Read the model definition and answer for the solid it produces. Units are mm, in the model's axes. A direction names the side the tool comes from. Coordinates: 2 decimals unless noted, no trailing zeros. Loops run counter-clockwise (first coordinate to the right, second up) from the corner with the lowest first, then second, coordinate; pieces in that order, holes last. Notation, with made-up numbers: (19.25, 14.25) -> (42.25, 14.25) arc R13 cw to (42.25, 20.25) -> close; hole circle Ø2 at (30.5, 49). An arc over 180 degrees is marked (long way). Answer as a JSON object with one key per item and string values. Group by question number.
Q1. Determine the mould class of faces 5 (the flat face through (25.441, 0, -11)), 6 (the cylindrical face through (-16.31, -20.796, 15.284)), 7 (the flat face through (137, -11.112, 9)) for opening direction X: released by +X, released by -X, zero draft, split by the parting line, or undercut.
Q2. Straight lines are drawn through the part: line 1 along Z through (x, y) = (0, 22); line 2 along X through (y, z) = (-24, -9); line 3 along X through (y, z) = (-17, 0.5). For each, find the intervals that lie inside material, in ascending order. Write a range as [from, to].
Q3. The part is cut by section B-B on z = -4. Write down the section's boundary in (x, y), and give its area (3 significant figures).
Q4. The part is cut by section D-D on z = -20. Write down the section's boundary in (x, y), and give its area (3 significant figures).
Q5. The part is cut by section C-C on y = 21.5. Write down the section's boundary in (x, z), and give its area (3 significant figures).
Q6. Each of these flat-tipped pins is pushed along its axis until it touches: P1, Ø10, axis at y = -17.5, z = -6, coming from the -X side; P2, Ø24.5, axis at y = -1.5, z = -16.5, coming from the -X side; P3, Ø3, axis at y = -16.5, z = 17.5, coming from the -X side; P4, Ø15, axis at x = 0, z = 0, coming from the +Y side. Where does it stop, or does it pass through?
Q7. The part is cut by section A-A on y = -13.5. Write down the section's boundary in (x, z).
Q8. For faces 1 (the flat face through (12, -11.163, -5)), 2 (the flat face through (107, 6, 0)), 3 (the flat face through (112.166, -21, -11)), 4 (the flat face through (150.089, -21, 11)), determine the directions among +Z, -Z, +X, -X, +Y, -Y from which every point of the face is accessible in a straight line to the end or side of a thin tool.
from build123d import *

# Parameters (mm, degrees)
F0_R      = 12.7
F1_DEPTH  = 30.1625
F3_R      = 3.302
F4_R      = 7.874
F5_DEPTH  = 19.05
F6_DEPTH  = 19.05
F7_R      = 3.302
F8_R      = 12.7
F9_DEPTH  = 11.1633
F11_DEPTH = 22.352


with BuildPart() as f1:
    # F0 (on Front) → F1 (new body, symmetric)
    with BuildSketch(Plane.XZ):
        with BuildLine():
            Line((194.2084, 0), (22.352, 0))
            ThreePointArc((22.352, 0), (-15.805251, 15.805251), (0, -22.352))
            Line((0, -22.352), (194.2084, -22.352))
            Line((194.2084, -22.352), (194.2084, 0))
        make_face()
        Circle(F0_R, mode=Mode.SUBTRACT)
    extrude(amount=F1_DEPTH, both=True)

    # F3
    f3_edges = [f1.edges().sort_by_distance(p)[0] for p in [
        (22.352, 0, 0),
    ]]
    fillet(f3_edges, radius=F3_R)

    # F4
    f4_edges = [f1.edges().sort_by_distance(p)[0] for p in [
        (194.2084, 0, 0),
    ]]
    fillet(f4_edges, radius=F4_R)

    # F2 (on face) → F5 (cut)
    with BuildSketch(Plane.XZ.offset(30.1625)):
        Polygon((112.1664, 0), (85.852, 0), (91.8464, -22.352), (112.1664, -22.352), align=None)
    extrude(amount=-F5_DEPTH, mode=Mode.SUBTRACT)

    # F2 (on face) → F6 (join)
    with BuildSketch(Plane.XZ.offset(30.1625)):
        with BuildLine():
            ThreePointArc((131.0386, 22.352), (123.246252, 9.78815), (112.1664, 0))
            Line((112.1664, 0), (131.0386, 0))
            Line((131.0386, 0), (150.0886, 0))
            Line((150.0886, 0), (150.0886, 22.352))
            Line((150.0886, 22.352), (131.0386, 22.352))
        make_face()
    extrude(amount=-F6_DEPTH)

    # F7
    f7_edges = [f1.edges().sort_by_distance(p)[0] for p in [
        (150.0886, -20.6375, 0),
        (150.0886, -20.6375, 22.352),
    ]]
    fillet(f7_edges, radius=F7_R)

    # F8 (on Front) → F9 (cut, symmetric)
    with BuildSketch(Plane.XZ):
        with BuildLine():
            ThreePointArc((25.440608, 0), (23.261179, 0.821417), (22.166074, 2.87699))
            ThreePointArc((22.166074, 2.87699), (-16.791641, 14.753058), (0, -22.352))
            Line((0, -22.352), (25.440608, -22.352))
            Line((25.440608, -22.352), (25.440608, 0))
        make_face()
        Circle(F8_R, mode=Mode.SUBTRACT)
    extrude(amount=F9_DEPTH, both=True, mode=Mode.SUBTRACT)

    # F10 (on face) → F11 (cut)
    with BuildSketch(Plane.XY):
        with BuildLine():
            ThreePointArc((161.6964, 7.8105), (159.836528, 12.300628), (155.3464, 14.1605))
            ThreePointArc((155.3464, 14.1605), (150.856272, 3.320372), (161.6964, 7.8105))
        make_face()
    extrude(amount=-F11_DEPTH, mode=Mode.SUBTRACT)


solid = f1.part
Final values:
{
 "1": {"face 5": "released by -X", "face 6": "undercut", "face 7": "zero draft"},
 "2": {"line 1": "z = [-22.35, -12.7], [12.7, 22.35]", "line 2": "x = [-20.46, -8.96], [8.96, 88.27], [112.17, 194.21]", "line 3": "x = [-22.35, -12.69], [12.69, 23.69], [112.92, 151.64]"},
 "3": {"outline": "(-21.99, -30.16) -> (-12.05, -30.16) -> (-12.05, -11.16) -> (-21.99, -11.16) -> close; (-21.99, 11.16) -> (-12.05, 11.16) -> (-12.05, 30.16) -> (-21.99, 30.16) -> close; (12.05, -30.16) -> (86.92, -30.16) -> (86.92, -11.11) -> (112.17, -11.11) -> (112.17, -30.16) -> (193.19, -30.16) -> (193.19, 30.16) -> (12.05, 30.16) -> (12.05, 11.16) -> (25.44, 11.16) -> (25.44, -11.16) -> (12.05, -11.16) -> close; hole circle Ø12.7 at (155.35, 7.81)", "area": "10,400 mm2"},
 "4": {"outline": "(-9.98, -30.16) -> (91.22, -30.16) -> (91.22, -11.11) -> (112.17, -11.11) -> (112.17, -30.16) -> (194.21, -30.16) -> (194.21, 30.16) -> (-9.98, 30.16) -> (-9.98, 11.16) -> (25.44, 11.16) -> (25.44, -11.16) -> (-9.98, -11.16) -> close; hole circle Ø12.7 at (155.35, 7.81)", "area": "11,000 mm2"},
 "5": {"outline": "(0, -22.35) -> (194.21, -22.35) -> (194.21, -7.87) arc R7.87 ccw to (186.33, 0) -> (25.44, 0) arc R3.3 cw to (22.17, 2.88) arc R22.35 ccw (long way) to start; hole circle Ø25.4 at (0, 0)", "area": "5,000 mm2"},
 "6": {"P1": "stops at x = -22.33", "P2": "stops at x = -20.47", "P3": "stops at x = -15.61", "P4": "passes through"},
 "7": {"outline": "(0, -22.35) -> (91.85, -22.35) -> (85.85, 0) -> (25.44, 0) arc R3.3 cw to (22.17, 2.88) arc R22.35 ccw (long way) to start; (112.17, -22.35) -> (194.21, -22.35) -> (194.21, -7.87) arc R7.87 ccw to (186.33, 0) -> (153.39, 0) arc R3.3 cw to (150.09, 3.3) -> (150.09, 19.05) arc R3.3 ccw to (146.79, 22.35) -> (131.04, 22.35) arc R50.8 cw to (112.17, 0) -> close; hole circle Ø25.4 at (0, 0)"},
 "8": {"face 1": "+Z, -Z, -X", "face 2": "+Z, +Y", "face 3": "+Z, -Z, -Y", "face 4": "+Z, +X, +Y, -Y"}
}
